```python
from build123d import *

# Parameters (mm, degrees)
SKETCH1_W           = 36.5
SKETCH1_H           = 110
BOSS_EXTRUDE1_DEPTH = 15
BOSS_EXTRUDE2_DEPTH = 15
FILLET1_R           = 10
FILLET2_R           = 5
SKETCH3_W           = 10
SKETCH3_H           = 15
BOSS_EXTRUDE3_DEPTH = 15
SKETCH4_R           = 2
CUT_EXTRUDE1_DEPTH  = 71.661605558


with BuildPart() as part:
    # Sketch1 → Boss-Extrude1 (new body)
    with BuildSketch(Plane(origin=(0, 0, 0), x_dir=(1, 0, 0), z_dir=(0, 1, 0))):
        Rectangle(SKETCH1_W, SKETCH1_H)
    extrude(amount=BOSS_EXTRUDE1_DEPTH)

    # Sketch2 → Boss-Extrude2 (add)
    with BuildSketch(Plane(origin=(0, 15, 0), x_dir=(1, 0, 0), z_dir=(0, 1, 0))):
        Polygon((-18.25, 11.5), (-41.75, 35), (-41.75, 55), (-18.25, 55), align=None)
    extrude(amount=-BOSS_EXTRUDE2_DEPTH)

    # Fillet1
    fillet1_edges = [part.edges().sort_by_distance(p)[0] for p in [
        (-18.25, 7.5, -11.5),
        (-41.75, 7.5, -35),
    ]]
    fillet(fillet1_edges, radius=FILLET1_R)

    # Fillet2
    fillet2_edges = [part.edges().sort_by_distance(p)[0] for p in [
        (-18.25, 7.5, 55),
    ]]
    fillet(fillet2_edges, radius=FILLET2_R)

    # Sketch3 → Boss-Extrude3 (add)
    with BuildSketch(Plane(origin=(0, 15, 0), x_dir=(1, 0, 0), z_dir=(0, 1, 0))):
        with Locations((23.25, -47.5)):
            Rectangle(SKETCH3_W, SKETCH3_H)
        with Locations((23.25, 47.5)):
            Rectangle(SKETCH3_W, SKETCH3_H)
    extrude(amount=-BOSS_EXTRUDE3_DEPTH)

    # Sketch4 → Cut-Extrude1 (cut, through all)
    with BuildSketch(Plane(origin=(0, 15, 0), x_dir=(1, 0, 0), z_dir=(0, 1, 0))):
        with Locations((18.957106781, 39.292893219)):
            Circle(SKETCH4_R)
        with Locations((18.957106781, -39.292893219)):
            Circle(SKETCH4_R)
    extrude(amount=-CUT_EXTRUDE1_DEPTH, mode=Mode.SUBTRACT)


solid = part.part
```
Check sheet for the modelled part. Datum: model origin and axes. Units: mm. A direction names the side the tool comes from. Give positions to 0.01 mm unless a question says otherwise; leave off trailing zeros. Write each loop counter-clockwise with the first axis right and the second up, starting at its lowest first coordinate (ties: lowest second). Pieces come first, ordered by that corner, then holes.
Item 1: Gauge pin test, flat ends, axial feed: pin 1 (1.5 mm diameter, centred on y = 7, z = 5, fed in from -X); pin 2 (6 mm diameter, centred on y = 11, z = -21, fed in from +X); pin 3 (3 mm diameter, centred on x = 18.96, z = -39.29, fed in from +Y); pin 4 (3 mm diameter, centred on x = -30.5, z = -29, fed in from -Y). Record the tip position at first contact, or that the pin passes through.
Item 2: Cross-section at C-C (z = 5.5). Enter the section's corners in (x, y).
Item 3: Scan lines: L1, parallel to Z at x = 19, y = 3.75; L2, parallel to X at y = 2.5, z = 21; L3, parallel to Z at x = -13.5, y = 7.75. Record each from-to range of solid material in increasing order.
Item 4: Access from +Z, -Z, +X, -X, +Y, -Y to the whole of each face (thin tool, end or side, straight path). Record for faces 4 (the face through (7, 8, 55)), 5 (the face through (-18.25, 7, 22)), 6 (the face through (18.25, 7, 1)).
Item 5: Cross-section at B-B (x = -23). Enter the section's corners in (y, z).
Item 6: Draft check along Z on faces 1 (the face through (24, 8, -40)), 2 (the face through (-29.88, 7.6, -23.13)), 3 (the face through (28.25, 8, 48)). Enter one of: released by +Z, released by -Z, zero draft, split by the parting line, or undercut.
Item 7: Cross-section at A-A (y = 10.75). Enter the section's corners in (x, z).
Report:
1. pin 1: stops at x = -18.25
1. pin 2: stops at x = 18.25
1. pin 3: passes through
1. pin 4: stops at y = 0
2. outline: (-18.25, 0) - (18.25, 0) - (18.25, 15) - (-18.25, 15) - close
3. L1: z = -55 to -41.29, 41.29 to 55
3. L2: x = -18.25 to 18.25
3. L3: z = -55 to 54.99
4. face 4: +Z, +X, -X, +Y, -Y
4. face 5: +Z, -X, +Y, -Y
4. face 6: +X, +Y, -Y
5. outline: (0, -55) - (15, -55) - (15, -16.25) - (0, -16.25) - close
6. face 1: undercut
6. face 2: released by +Z
6. face 3: zero draft
7. outline: (-41.75, -55) - (28.25, -55) - (28.25, -40) - (20.83, -40) arc R2 cw (long way) to (18.25, -37.42) - (18.25, 37.42) arc R2 cw (long way) to (20.83, 40) - (28.25, 40) - (28.25, 55) - (-13.25, 55) arc R5 ccw to (-18.25, 50) - (-18.25, -7.36) arc R10 cw to (-21.18, -14.43) - (-38.82, -32.07) arc R10 ccw to (-41.75, -39.14) - close
